Input: dimensioned drawing with shaded views. Units: mm. Origin: part minimum x, y, z. A direction names the side the tool comes from. Give positions to 0.01 mm unless a question says otherwise; leave off trailing zeros. Order: outer loops, then holes, each group sorted by start corner. A loop starts at its lowest first (then second) coordinate and runs counter-clockwise, first axis right, second up. Notation, with made-up numbers: (80, -28) -> (85, -28) arc R18 cw to (85, -17) -> close; hole circle Ø11 at (27, 53). An arc over 180 degrees is marked (long way). One line per question, with ' | ' between items. Start each with the question number.
(1) Ray query, L1, parallel to X at y = 36.5, z = 38.5; L2, parallel to Y at x = 5.65, z = 15.5; L3, parallel to X at y = 3.5, z = 30. Return the intervals inside material, ascending.
(2) Section A-A (x = 5.65). Return loops of the section in (y, z).
(3) Section D-D (y = 32.5). Return loops of the section in (x, z).
(4) First-contact query: pin 1 Ø2 at (y, z) = (18, 47) entering from +X; pin 2 Ø2 at (y, z) = (17.5, 21.5) entering from +X; pin 3 Ø8 at (x, y) = (36.65, 5.65) entering from +Z. Flat tips, straight axial feed; report the tip coordinate or a pass-through.
(5) Mould query, pull axis Z, two halves, no side actions, for the marked faces 1, 2 and 3. Classes: +Z half, -Z half, draft (parallel to the pull), parting line (faces both ways), or undercut.
(6) Section C-C (z = 35). Return loops of the section in (x, y), then the cut area to 3 significant figures.
(7) Set-up query: the marked faces 4, 5, 6 and 7. Return all of +Z, -Z, +X, -X, +Y, -Y with unobstructed straight access to the full face (end or side cutting, diameter ignored); none if empty.
(8) Section B-B (y = 5.65). Return loops of the section in (x, z).
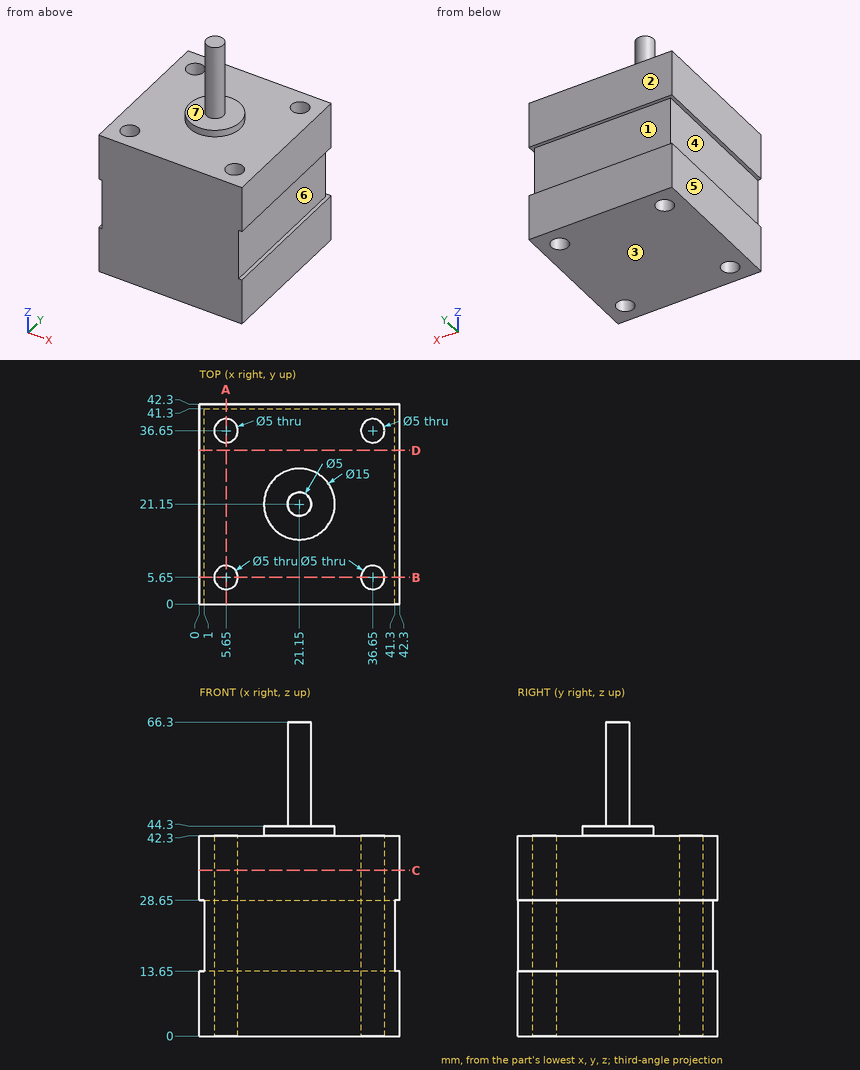
Response:
1) L1: x = 0 to 3.15, 8.15 to 34.15, 39.15 to 42.3 | L2: y = 0 to 3.15, 8.15 to 34.15, 39.15 to 41.3 | L3: x = 0 to 4.37, 6.93 to 35.37, 37.93 to 42.3
2) outline: (0, 0) -> (3.15, 0) -> (3.15, 42.3) -> (0, 42.3) -> close; (8.15, 0) -> (34.15, 0) -> (34.15, 42.3) -> (8.15, 42.3) -> close; (39.15, 0) -> (42.3, 0) -> (42.3, 13.65) -> (41.3, 13.65) -> (41.3, 28.65) -> (42.3, 28.65) -> (42.3, 42.3) -> (39.15, 42.3) -> close
3) outline: (0, 0) -> (42.3, 0) -> (42.3, 13.65) -> (41.3, 13.65) -> (41.3, 28.65) -> (42.3, 28.65) -> (42.3, 42.3) -> (0, 42.3) -> (0, 28.65) -> (1, 28.65) -> (1, 13.65) -> (0, 13.65) -> close
4) pin 1: stops at x = 22.43 | pin 2: stops at x = 41.3 | pin 3: stops at z = 42.3
5) face 1: undercut | face 2: draft | face 3: -Z half
6) outline: (0, 0) -> (42.3, 0) -> (42.3, 42.3) -> (0, 42.3) -> close; hole circle Ø5 at (5.65, 5.65); hole circle Ø5 at (5.65, 36.65); hole circle Ø5 at (36.65, 5.65); hole circle Ø5 at (36.65, 36.65) | area: 1,710 mm^2
7) face 4: -X, +Y, -Y | face 5: +Z, -Z, -X, +Y, -Y | face 6: +X, +Y, -Y | face 7: +Z
8) outline: (0, 0) -> (3.15, 0) -> (3.15, 42.3) -> (0, 42.3) -> (0, 28.65) -> (1, 28.65) -> (1, 13.65) -> (0, 13.65) -> close; (8.15, 0) -> (34.15, 0) -> (34.15, 42.3) -> (8.15, 42.3) -> close; (39.15, 0) -> (42.3, 0) -> (42.3, 13.65) -> (41.3, 13.65) -> (41.3, 28.65) -> (42.3, 28.65) -> (42.3, 42.3) -> (39.15, 42.3) -> close
